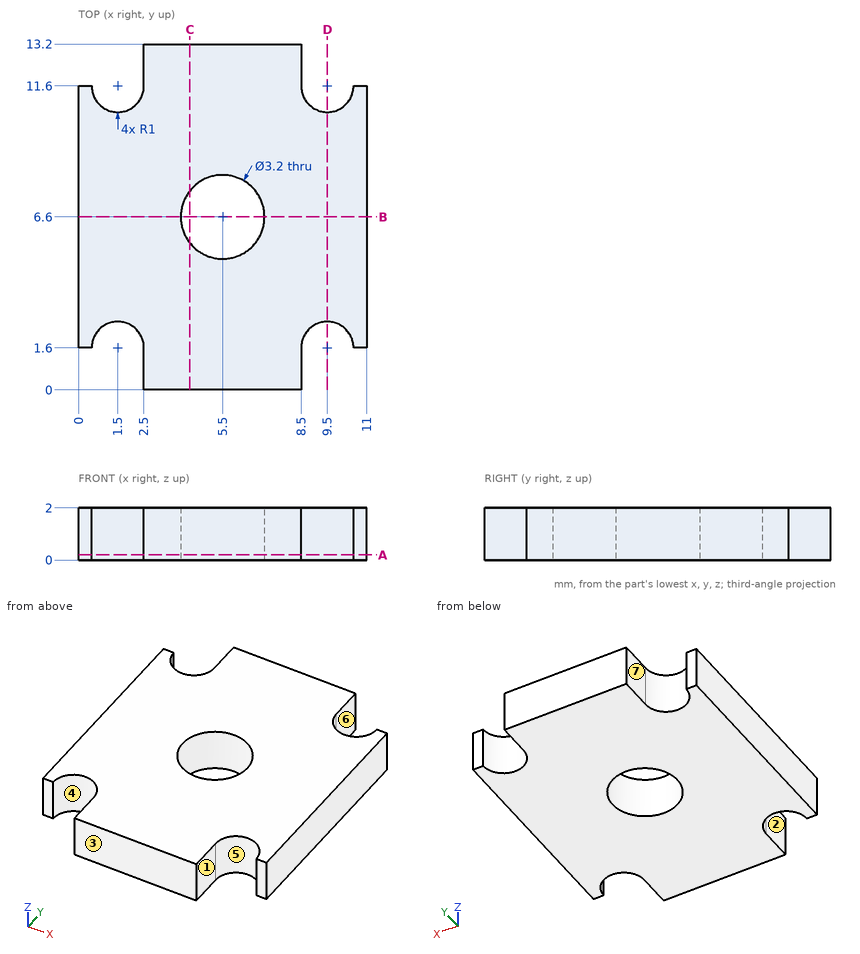
Drawing for the job (mm, zero at the part's lowest x, y, z). A direction names the side the tool comes from. Round coordinates to 2 decimals unless told otherwise and drop trailing zeros. Loops run counter-clockwise (first coordinate to the right, second up) from the corner with the lowest first, then second, coordinate; pieces in that order, holes last. Notation, with made-up numbers: (43, 74.25) -> (71, 74.25) arc R25 ccw to (71, 105.25) -> close; hole circle Ø4 at (-15.5, 1.5). An arc over 180 degrees is marked (long way). Answer as CSV lines item,"result". Start each with the question number.
1) Slice it at C-C (x = 4.25). List the corners of the cut face in (y, z), plus the area to 3 significant figures.
2) Slice it at A-A (z = 0.2). List the corners of the cut face in (x, y).
3) Probe line 1 along X through (y, z) = (2.25, 0.4); line 2 along Y through (x, z) = (5.5, 0.5); line 3 along X through (y, z) = (2, 1.7). List the from-to ranges inside material, lowest first.
4) Mould opens along X. For the marked faces 4, 5, 6 and 7 say: +X half, -X half, draft (parallel to the pull), parting line (faces both ways), or undercut.
5) Pin check, flat tips, straight feed: P1, Ø0.5, axis at y = 12, z = 1, coming from the +X side; P2, Ø0.8, axis at y = 1, z = 1, coming from the -X side; P3, Ø0.6, axis at x = 0, z = 1.5, coming from the +Y side. Stop position of each tip, or through.
6) Slice it at D-D (x = 9.5). List the corners of the cut face in (y, z).
7) Slice it at B-B (y = 6.6). List the corners of the cut face in (x, z).
8) Tool access for the marked faces 1, 2 and 3: list every direction of +Z, -Z, +X, -X, +Y, -Y with a clear straight run to the whole face (end or side of a thin tool).
Filled in:
1,outline,"(0, 0) -> (5.6, 0) -> (5.6, 2) -> (0, 2) -> close; (7.6, 0) -> (13.2, 0) -> (13.2, 2) -> (7.6, 2) -> close"
1,area,"22.4 mm2"
2,outline,"(0, 1.6) -> (0.5, 1.6) arc R1 cw to (2.5, 1.6) -> (2.5, 0) -> (8.5, 0) -> (8.5, 1.6) arc R1 cw to (10.5, 1.6) -> (11, 1.6) -> (11, 11.6) -> (10.5, 11.6) arc R1 cw to (8.5, 11.6) -> (8.5, 13.2) -> (2.5, 13.2) -> (2.5, 11.6) arc R1 cw to (0.5, 11.6) -> (0, 11.6) -> close; hole circle Ø3.2 at (5.5, 6.6)"
3,line 1,"x = 0 to 0.74, 2.26 to 8.74, 10.26 to 11"
3,line 2,"y = 0 to 5, 8.2 to 13.2"
3,line 3,"x = 0 to 0.58, 2.42 to 8.58, 10.42 to 11"
4,face 4,"undercut"
4,face 5,"undercut"
4,face 6,"+X half"
4,face 7,"-X half"
5,P1,"stops at x = 8.5"
5,P2,"stops at x = 2.5"
5,P3,"stops at y = 11.6"
6,outline,"(2.6, 0) -> (10.6, 0) -> (10.6, 2) -> (2.6, 2) -> close"
7,outline,"(0, 0) -> (3.9, 0) -> (3.9, 2) -> (0, 2) -> close; (7.1, 0) -> (11, 0) -> (11, 2) -> (7.1, 2) -> close"
8,face 1,"+Z, -Z, +X, -Y"
8,face 2,"+Z, -Z, -X, -Y"
8,face 3,"+Z, -Z, +X, -X, -Y"
